from build123d import *

# Parameters (mm, degrees)
SKETCH1_R           = 3
SKETCH1_R_2         = 1.5
BOSS_EXTRUDE1_DEPTH = 40
SKETCH2_R           = 22.5
SKETCH2_R_2         = 1.5
BOSS_EXTRUDE2_DEPTH = 3
BOSS_EXTRUDE4_DEPTH = 10


with BuildPart() as part:
    # Sketch1 → Boss-Extrude1 (new body)
    with BuildSketch(Plane(origin=(0, 0, 0), x_dir=(0, 0, -1), z_dir=(1, 0, 0))):
        Circle(SKETCH1_R)
        Circle(SKETCH1_R_2, mode=Mode.SUBTRACT)
    extrude(amount=BOSS_EXTRUDE1_DEPTH)

    # Sketch2 → Boss-Extrude2 (add)
    with BuildSketch(Plane(origin=(40, 0, 0), x_dir=(0, 0, -1), z_dir=(1, 0, 0))):
        Circle(SKETCH2_R)
        Circle(SKETCH2_R_2, mode=Mode.SUBTRACT)
    boss_extrude2 = extrude(amount=BOSS_EXTRUDE2_DEPTH)

    # Mirror1: Boss-Extrude2 across plane
    add(boss_extrude2.mirror(Plane(origin=(20, 0, 0), x_dir=(0, 0, 1), z_dir=(1, 0, 0))))

    # Sketch4 → Boss-Extrude4 (add)
    with BuildSketch(Plane.ZY.offset(3)):
        with BuildLine():
            Line((-1, 1.118033989), (-1, -1.118033989))
            ThreePointArc((-1, -1.118033989), (-1.5, 0), (-1, 1.118033989))
        make_face()
    extrude(amount=-BOSS_EXTRUDE4_DEPTH)


solid = part.part
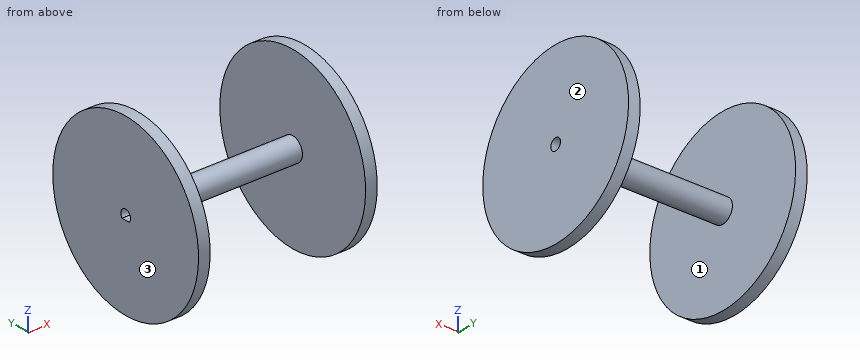
The listing builds one solid part. Answer for the finished solid, in the listing's coordinates (mm). Face numbers are marked on the shaded views. Round coordinates to 2 decimals unless told otherwise and drop trailing zeros. Write each loop counter-clockwise with the first axis right and the second up, starting at its lowest first coordinate (ties: lowest second). Pieces come first, ordered by that corner, then holes. Notation, with made-up numbers: M -16,28 L 36,28 A20 ccw 36,33 Z; hole C 76.5,-31 d7. An arc over 180 degrees is marked long. Write each question's results on one line, items separated by ' | '. Start each with the question number.
Item 1: The mould has two halves that part along X. Classify the marked faces 1, 2 and 3: +X half, -X half, draft (parallel to the pull), parting line (faces both ways), or undercut.
Item 2: Find section B-B on z = 0. Write down the section's boundary in (x, y), and give its area (3 significant figures).
Item 3: Given pin 1 Ø10 at (x, y) = (36, -9) entering from -Z; pin 2 Ø5 at (x, z) = (10, -4.5) entering from -Y; pin 3 Ø10 at (x, z) = (23.5, 3.5) entering from +Y, each flat-ended and moving along its own axis, determine where each tip first touches the part or whether it passes through.
Item 4: Find section C-C on x = 9.5. Write down the section's boundary in (y, z).
Item 5: Find section A-A on y = -13.5. Write down the section's boundary in (x, z), and give its area (3 significant figures).
Item 6: Find section D-D on y = 0. Write down the section's boundary in (x, z), and give its area (3 significant figures).
Item 7: Straight lines are drawn through the part: probe 1 along X at (y, z) = (-12.5, -4.5); probe 2 along Y at (x, z) = (15.5, 0); probe 3 along Y at (x, z) = (3, 1). For each, find the intervals that lie inside material, in ascending order.
Answer block:
1) face 1: undercut | face 2: +X half | face 3: -X half
2) outline: M -3,-22.5 L 0,-22.5 L 0,-3 L 40,-3 L 40,-22.5 L 43,-22.5 L 43,-1.5 L -3,-1.5 Z; M -3,1.5 L 43,1.5 L 43,22.5 L 40,22.5 L 40,3 L 0,3 L 0,22.5 L -3,22.5 Z | area: 372 mm²
3) pin 1: stops at z = -21.69 | pin 2: stops at y = -2.24 | pin 3: stops at y = 3
4) outline: C 0,0 d6; hole C 0,0 d3
5) outline: M -3,-18 L 0,-18 L 0,18 L -3,18 Z; M 40,-18 L 43,-18 L 43,18 L 40,18 Z | area: 216 mm²
6) outline: M -3,-22.5 L 0,-22.5 L 0,-3 L 40,-3 L 40,-22.5 L 43,-22.5 L 43,-1.5 L 7,-1.5 L 7,-1 L -3,-1 Z; M -3,1.5 L 43,1.5 L 43,22.5 L 40,22.5 L 40,3 L 0,3 L 0,22.5 L -3,22.5 Z | area: 377 mm²
7) probe 1: x = -3 to 0, 40 to 43 | probe 2: y = -3 to -1.5, 1.5 to 3 | probe 3: y = -2.83 to -1.12, 1.12 to 2.83
